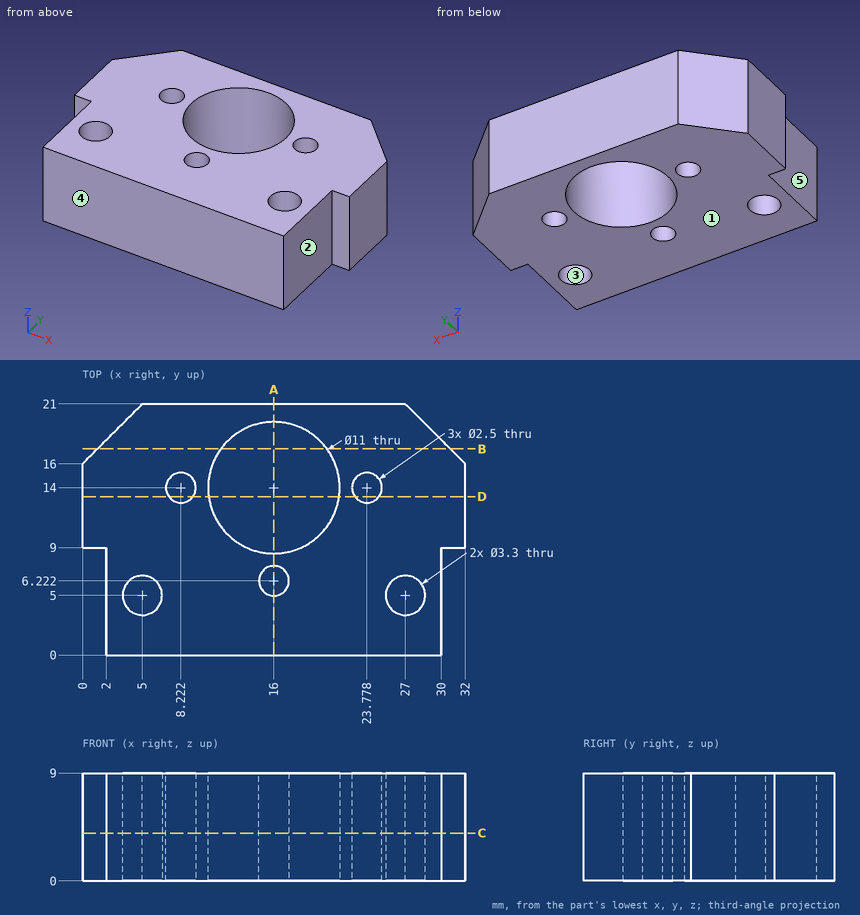
Geometry check sheet. Reference: drawing and pictorial views, mm from the part's lowest x, y, z. A direction names the side the tool comes from. Round coordinates to 2 decimals unless told otherwise and drop trailing zeros. Loops run counter-clockwise (first coordinate to the right, second up) from the corner with the lowest first, then second, coordinate; pieces in that order, holes last. Notation, with made-up numbers: (-27, 18.25) -> (6, 18.25) arc R25 ccw to (6, 42.25) -> close; hole circle Ø9 at (-31.75, -39.75). An arc over 180 degrees is marked (long way). Use a Markdown table: item, result.
(1) Sectioned sample at D-D (y = 13.25). Enter the section's corners in (x, z), then the cut area to 3 significant figures.
Calculated:
| item | result |
|---|---|
| outline | (0, 0) -> (7.22, 0) -> (7.22, 9) -> (0, 9) -> close; (9.22, 0) -> (10.55, 0) -> (10.55, 9) -> (9.22, 9) -> close; (21.45, 0) -> (22.78, 0) -> (22.78, 9) -> (21.45, 9) -> close; (24.78, 0) -> (32, 0) -> (32, 9) -> (24.78, 9) -> close |
| area | 154 mm² |
(2) Mould release check, pull along X, two halves, no side actions. Record for the marked faces 3, 4 and 5: released by +X, released by -X, zero draft, split by the parting line, or undercut.
Calculated:
| item | result |
|---|---|
| face 3 | undercut |
| face 4 | zero draft |
| face 5 | released by -X |
(3) Sectioned sample at C-C (z = 4). Enter the section's corners in (x, y), then the cut area to 3 significant figures.
Calculated:
| item | result |
|---|---|
| outline | (0, 9) -> (2, 9) -> (2, 0) -> (30, 0) -> (30, 9) -> (32, 9) -> (32, 16) -> (27, 21) -> (5, 21) -> (0, 16) -> close; hole circle Ø3.3 at (5, 5); hole circle Ø2.5 at (8.22, 14); hole circle Ø11 at (16, 14); hole circle Ø2.5 at (16, 6.22); hole circle Ø2.5 at (23.78, 14); hole circle Ø3.3 at (27, 5) |
| area | 484 mm² |
(4) Set-up check for the marked faces 1 and 2: record each of +Z, -Z, +X, -X, +Y, -Y from which the full face is reachable in a straight line by a thin tool's end or side.
Calculated:
| item | result |
|---|---|
| face 1 | -Z, +X, -X, +Y, -Y |
| face 2 | +Z, -Z, +X, -Y |
(5) Go/stop test with flat-tipped pins: P1, Ø4.5, axis at x = 27, y = 5, coming from the +Z side; P2, Ø2.5, axis at y = 6, z = 3, coming from the -X side. Record where each tip stops, or that it passes through.
Calculated:
| item | result |
|---|---|
| P1 | z = 9 |
| P2 | x = 2 |
(6) Sectioned sample at A-A (x = 16). Enter the section's corners in (y, z).
Calculated:
| item | result |
|---|---|
| outline | (0, 0) -> (4.97, 0) -> (4.97, 9) -> (0, 9) -> close; (7.47, 0) -> (8.5, 0) -> (8.5, 9) -> (7.47, 9) -> close; (19.5, 0) -> (21, 0) -> (21, 9) -> (19.5, 9) -> close |
(7) Sectioned sample at B-B (y = 17.25). Enter the section's corners in (x, z).
Calculated:
| item | result |
|---|---|
| outline | (1.25, 0) -> (11.56, 0) -> (11.56, 9) -> (1.25, 9) -> close; (20.44, 0) -> (30.75, 0) -> (30.75, 9) -> (20.44, 9) -> close |
(8) Scan lines: probe 1 along X at (y, z) = (6, 4.5); probe 2 along X at (y, z) = (5.25, 0.5) (1 decimal); probe 3 along Y at (x, z) = (27, 4). Record each from-to range of solid material in increasing order.
Calculated:
| item | result |
|---|---|
| probe 1 | 2 to 3.69, 6.31 to 14.77, 17.23 to 25.69, 28.31 to 30 |
| probe 2 | 2 to 3.4, 6.6 to 15.2, 16.8 to 25.4, 28.6 to 30 |
| probe 3 | 0 to 3.35, 6.65 to 21 |
